Autodesk Inventor part; units mm, degrees
ref_plane "YZ Plane" through (0, 0, 0) normal (1, 0, 0) x (0, 1, 0)
ref_plane "XZ Plane" through (0, 0, 0) normal (0, 1, 0) x (-1, 0, 0)
ref_plane "XY Plane" through (0, 0, 0) normal (0, 0, 1) x (1, 0, 0)
sketch "Sketch2" plane through (0, 0, 0) normal (0, 0, 1) x (1, 0, 0)
  line L0 (0, 0) -> (55, 0)
  line L1 (55, 0) -> (55, 40)
  line L2 (55, 40) -> (0, 40)
  line L3 (0, 40) -> (0, 0)
  line L4 (35, 40) -> (35, 0)
  line L5 (20, 40) -> (20, 0)
  line L6 (0, 20) -> (55, 20) construction
  line L7 (27.5, 0) -> (27.5, 40) construction
  circle A0 centre (6.5, 20) radius 2
  circle A1 centre (48.5, 20) radius 2
  circle A2 centre (27.5, 7.5) radius 2.6
  circle A3 centre (27.5, 32.5) radius 2.6
  point P0 (27.5, 7.5)
  point P1 (6.5, 20)
  point P2 (27.5, 32.5)
  dimension "d19" = 55
  dimension "d20" = 40
  dimension "d21" = 20
  dimension "d23" = 6.5
  dimension "d24" = 7.5
  dimension "d25" = 4
  dimension "d26" = 5.2
extrude "Extrusion1" add sketch "Sketch2" against normal blind 10 contours L3 L2 L5 L0 | L5 L2 L4 L0 | L4 L2 L1 L0 | A0 | A1 | A2 | A3
extrude "Extrusion2" cut sketch "Sketch2" against normal blind 5 contours L5 L2 L4 L0
hole "Hole1" at (6.5, 20, 0) at (48.5, 20, 0) direction (0, 0, -1) diameter 4 end through all
hole "Hole2" at (27.5, 7.5, 0) at (27.5, 32.5, 0) direction (0, 0, -1) diameter 5.2 end through all
thread "Thread3"
thread "Thread4"
properties part number "Leadscrew Bearing Bracket" material "Stainless Steel"
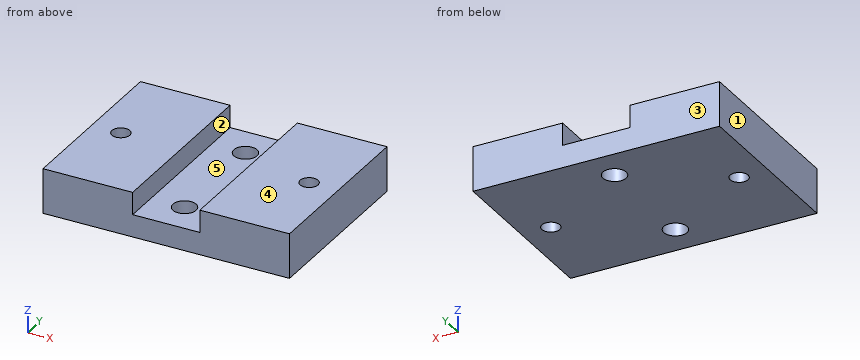
Verification items for the finished model (mm, model axes). Face numbers are marked on the shaded views. A direction names the side the tool comes from. Give positions to 0.01 mm unless a question says otherwise; leave off trailing zeros. Write each loop counter-clockwise with the first axis right and the second up, starting at its lowest first coordinate (ties: lowest second). Pieces come first, ordered by that corner, then holes. Notation, with made-up numbers: (-11, -37.75) -> (42, -37.75) arc R15 cw to (42, -33.75) -> close; hole circle Ø11 at (5, -4.75). An arc over 180 degrees is marked (long way). Use CSV: the item, a comma, the result in double quotes.
(1) Sectioned sample at A-A (z = -1.25). Record the cut outline in (x, y).
Derived:
outline,"(0, 0) -> (20, 0) -> (20, 40) -> (0, 40) -> close; (35, 0) -> (55, 0) -> (55, 40) -> (35, 40) -> close; hole circle Ø4 at (6.5, 20); hole circle Ø4 at (48.5, 20)"
(2) Set-up check for the marked faces 4 and 5: record each of +Z, -Z, +X, -X, +Y, -Y from which the full face is reachable in a straight line by a thin tool's end or side.
Derived:
face 4,"+Z, +X, -X, +Y, -Y"
face 5,"+Z, +Y, -Y"
(3) Material ranges on L1, parallel to X at y = 20, z = -3.25; L2, parallel to Y at x = 27.5, z = -8.85; L3, parallel to X at y = 20, z = -5.25, recorded low to high.
Derived:
L1,"x = 0 to 4.5, 8.5 to 20, 35 to 46.5, 50.5 to 55"
L2,"y = 0 to 4.9, 10.1 to 29.9, 35.1 to 40"
L3,"x = 0 to 4.5, 8.5 to 46.5, 50.5 to 55"
(4) Release check for a two-part mould opening along X. For the marked faces 1, 2 and 3 record: +X half, -X half, draft (parallel to the pull), parting line (faces both ways), or undercut.
Derived:
face 1,"-X half"
face 2,"undercut"
face 3,"draft"
(5) Go/stop test with a flat-tipped pin: pin 1 (8.5 mm diameter, centred on x = 27.5, y = 32.5, fed in from +Z). Record where the tip stops, or that it passes through.
Derived:
pin 1,"stops at z = -5"
(6) Sectioned sample at B-B (y = 7.5). Record the cut outline in (x, z).
Derived:
outline,"(0, -10) -> (24.9, -10) -> (24.9, -5) -> (20, -5) -> (20, 0) -> (0, 0) -> close; (30.1, -10) -> (55, -10) -> (55, 0) -> (35, 0) -> (35, -5) -> (30.1, -5) -> close"
(7) Sectioned sample at D-D (y = 20). Record the cut outline in (x, z), plus the area to 3 significant figures.
Derived:
outline,"(0, -10) -> (4.5, -10) -> (4.5, 0) -> (0, 0) -> close; (8.5, -10) -> (46.5, -10) -> (46.5, 0) -> (35, 0) -> (35, -5) -> (20, -5) -> (20, 0) -> (8.5, 0) -> close; (50.5, -10) -> (55, -10) -> (55, 0) -> (50.5, 0) -> close"
area,"395 mm^2"
(8) Sectioned sample at C-C (x = 48.5). Record the cut outline in (y, z).
Derived:
outline,"(0, -10) -> (18, -10) -> (18, 0) -> (0, 0) -> close; (22, -10) -> (40, -10) -> (40, 0) -> (22, 0) -> close"
